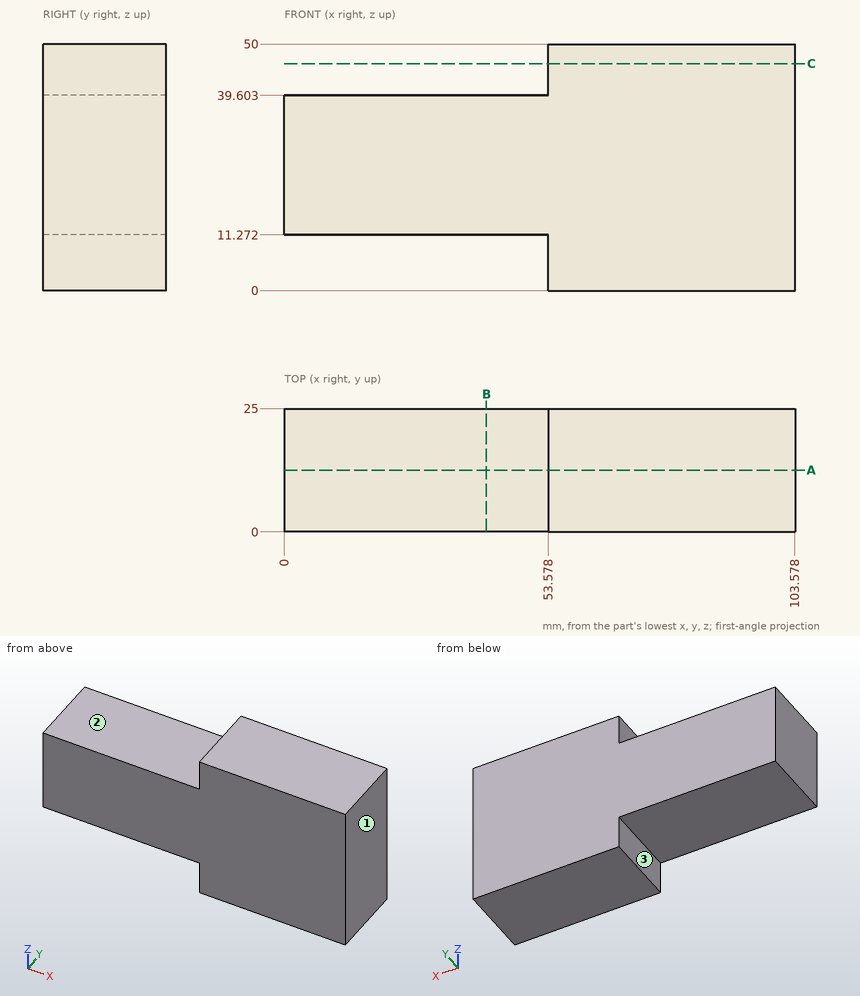
Design review of the part shown in the three views and the two pictorial views. Dimensions are in mm from the part's minimum x, y and z. A direction names the side the tool comes from. Give positions to 0.01 mm unless a question says otherwise; leave off trailing zeros. Loops run counter-clockwise (first coordinate to the right, second up) from the corner with the lowest first, then second, coordinate; pieces in that order, holes last. Notation, with made-up numbers: M -24.5,10.5 L 10.5,10.5 A5 cw 10.5,19.5 Z; hole C 88.25,30.5 d11. An arc over 180 degrees is marked long. Answer as a JSON object with one key per item and string values. Group by question number.
Q1. Add section C-C on z = 46. Give the boundary of the cut face in (x, y).
Q2. Tool access review of the marked faces 1, 2 and 3: name each direction out of +Z, -Z, +X, -X, +Y, -Y from which nothing blocks a thin tool from reaching the whole face with its end or side.
Q3. Add section A-A on y = 12.5. Give the boundary of the cut face in (x, z), and give its area (3 significant figures).
Q4. Add section B-B on x = 41. Give the boundary of the cut face in (y, z).
Q5. Insertion check: P1, Ø1, axis at x = 30, z = 37, coming from the -Y side; P2, Ø3.5, axis at y = 7, z = 3, coming from the -X side; P3, Ø12.5, axis at x = 30.5, y = 6.5, coming from the +Z side; P4, Ø1.5, axis at x = 43, y = 15, coming from the -Z side. Each pin has a flat end and moves straight along its axis. Give the tip position at first contact, or say it passes through.
Q6. For probe 1 along Z at (x, y) = (31, 7.75); probe 2 along X at (y, z) = (18.25, 40), list the stretches that pass through material, from the lowest coordinate up. Write a range as [from, to].
Checked values:
{
 "1": {"outline": "M 53.58,0 L 103.58,0 L 103.58,25 L 53.58,25 Z"},
 "2": {"face 1": "+Z, -Z, +X, +Y, -Y", "face 2": "+Z, -X, +Y, -Y", "face 3": "-Z, -X, +Y, -Y"},
 "3": {"outline": "M 0,11.27 L 53.58,11.27 L 53.58,0 L 103.58,0 L 103.58,50 L 53.58,50 L 53.58,39.6 L 0,39.6 Z", "area": "4,020 mm²"},
 "4": {"outline": "M 0,11.27 L 25,11.27 L 25,39.6 L 0,39.6 Z"},
 "5": {"P1": "y = 0", "P2": "x = 53.58", "P3": "z = 39.6", "P4": "z = 11.27"},
 "6": {"probe 1": "[11.27, 39.6]", "probe 2": "[53.58, 103.58]"}
}
